Can you work these out from the model? Positions are in its coordinate system, mm. A direction names the side the tool comes from. Coordinates: 2 decimals unless noted, no trailing zeros. Write each loop counter-clockwise with the first axis right and the second up, starting at its lowest first coordinate (ties: lowest second). Pieces come first, ordered by that corner, then holes. Notation, with made-up numbers: (52, 71.5) - (73, 71.5) arc R18 cw to (73, 105.5) - close; hole circle Ø5 at (-39, 72). An arc over 180 degrees is marked (long way). Use one line per item in the form item = value. Start each with the question number.
(1) On a 3-axis mill with a long thin cutter (end or side, diameter ignored), from which of +Z, -Z, +X, -X, +Y, -Y can I reach the whole of each face in a straight line? I mean faces 1 (the face through (-10, -11, 4)), 2 (the face through (-12, -11, 2.5)). Say none if no direction works.
(2) If we section it at C-C on x = -9.75: Please give me the cut outline in (y, z), then the cut area to 3 significant figures.
(3) If we section it at B-B on z = 4.4: Please give me the cut outline in (x, y).
(4) For pin 1 Ø1 at (x, z) = (-8.5, 5.5) entering from -Y; pin 2 Ø2 at (y, z) = (-12.5, 5) entering from +X; pin 3 Ø2.5 at (x, y) = (-7.5, -11) entering from -Z, each with a flat end and sliding along its axis, tell me the tip position at first contact or that it passes through.
(5) If we section it at A-A on y = -9: Please give me the cut outline in (x, z), then the cut area to 3 significant figures.
(6) If I drill on probe 1 along Z at (x, y) = (-9.25, -13.75); probe 2 along X at (y, z) = (-12.5, 4.85); probe 3 along X at (y, z) = (-11, 7.9), over which ranges is the centre line in solid material (lowest first)? Write a range as from..to.
```python
from build123d import *

# Parameters (mm, degrees)
BOX036_W                = 3
BOX036_H                = 8
BOX036_DEPTH            = 4
BOX035_W                = 8
BOX035_H                = 8
BOX035_DEPTH            = 2
CHAMFER_SIZE            = 1
CHAMFER_PLACEMENT_ANGLE = 180


with BuildPart() as cubo036:
    # Box036 → Box036 (new body)
    with BuildSketch(Plane(origin=(-13, -15, 2.5), x_dir=(1, 0, 0), z_dir=(0, 0, 1))):
        with Locations((1.5, 4)):
            Rectangle(BOX036_W, BOX036_H)
    extrude(amount=BOX036_DEPTH)


with BuildPart() as fusion002021:
    # Box035 → Box035 (new body)
    with BuildSketch(Plane(origin=(-13, -15, 6), x_dir=(1, 0, 0), z_dir=(0, 0, 1))):
        with Locations((4, 4)):
            Rectangle(BOX035_W, BOX035_H)
    extrude(amount=BOX035_DEPTH)

    # Chamfer
    chamfer_edges = [fusion002021.edges().sort_by_distance(p)[0] for p in [
        (-13, -11, 8),
    ]]
    chamfer(chamfer_edges, length=CHAMFER_SIZE)


with BuildPart() as fusion002021_1:
    # Chamfer placement: moved
    add(fusion002021.part.moved(Location((-18, -22, 0.5))).rotate(Axis((-18, -22, 0.5), (0, 0, 1)), CHAMFER_PLACEMENT_ANGLE))

    # Fusion002021: union Cubo036
    add(cubo036.part)


solid = fusion002021_1.part
```
Reported:
q1.face_1 = -Z, +X, +Y, -Y
q1.face_2 = -Z, +X, -X, +Y, -Y
q2.outline = (-15, 6.5) - (-7, 6.5) - (-7, 8.5) - (-15, 8.5) - close
q2.area = 16.0 mm2
q3.outline = (-13, -15) - (-10, -15) - (-10, -7) - (-13, -7) - close
q4.pin_1 = through
q4.pin_2 = -10
q4.pin_3 = 6.5
q5.outline = (-13, 2.5) - (-10, 2.5) - (-10, 6.5) - (-5, 6.5) - (-5, 7.5) - (-6, 8.5) - (-13, 8.5) - close
q5.area = 27.5 mm2
q6.probe_1 = 6.5..8.5
q6.probe_2 = -13..-10
q6.probe_3 = -13..-5.4
